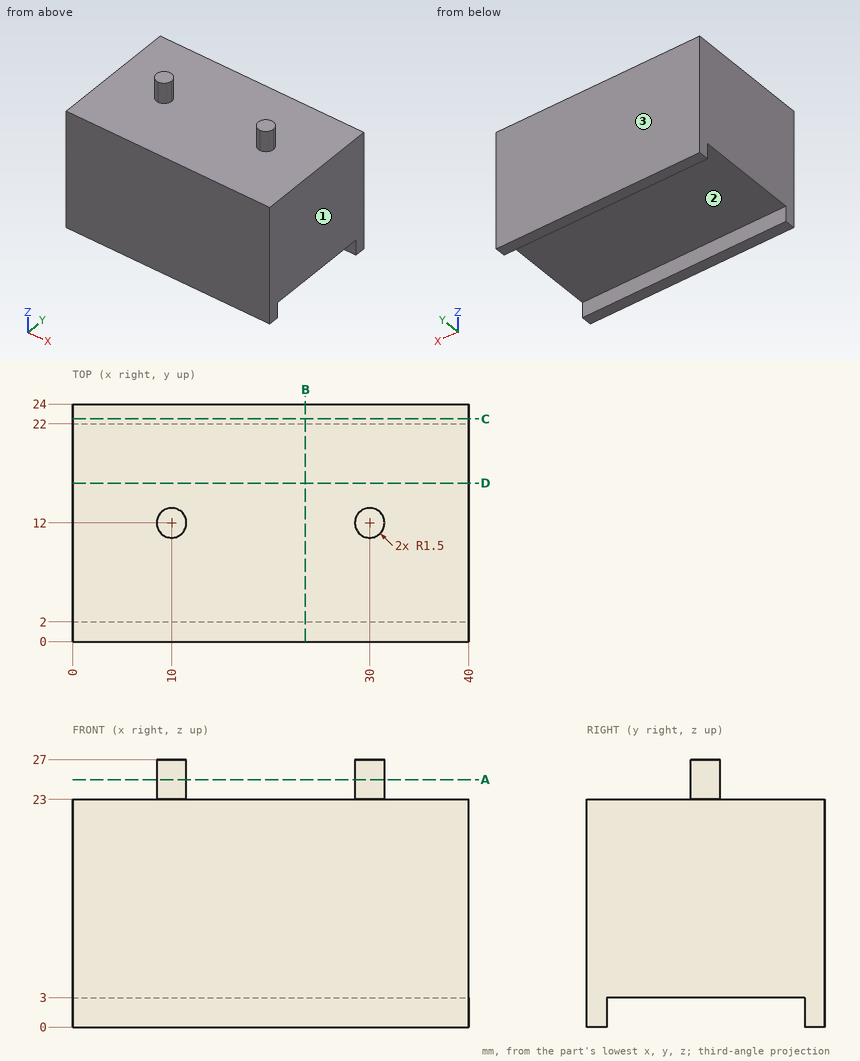
Drawing for the job (mm, zero at the part's lowest x, y, z). Round coordinates to 2 decimals unless told otherwise and drop trailing zeros. Write each loop counter-clockwise with the first axis right and the second up, starting at its lowest first coordinate (ties: lowest second). Pieces come first, ordered by that corner, then holes. Notation, with made-up numbers: (-14, -33) - (-9, -33) arc R12 cw to (-9, -26) - close; hole circle Ø8 at (-36.5, 51). An arc over 180 degrees is marked (long way). Return JSON: item names as keys, results as strings. Group by question number.
Item 1: Mould opens along Y. For the marked faces 1, 2 and 3 say: +Y half, -Y half, draft (parallel to the pull), parting line (faces both ways), or undercut.
Item 2: Flat gauge pins, fed straight in: pin 1 Ø1 at (x, y) = (30.5, 14) entering from +Z; pin 2 Ø3 at (x, z) = (33.5, 24) entering from +Y. Where does each tip first touch, or does it go through?
Item 3: Band-saw the part on A-A on z = 25. List the corners of the cut face in (x, y).
Item 4: Band-saw the part on D-D on y = 16. List the corners of the cut face in (x, z).
Item 5: Probe probe 1 along Z at (x, y) = (7, 5). List the from-to ranges inside material, lowest first.
Item 6: Band-saw the part on C-C on y = 22.5. List the corners of the cut face in (x, z).
Item 7: Band-saw the part on B-B on x = 23.5. List the corners of the cut face in (y, z).
Resolved:
{
 "1": {"face 1": "draft", "face 2": "undercut", "face 3": "+Y half"},
 "2": {"pin 1": "stops at z = 23", "pin 2": "stops at y = 24"},
 "3": {"outline": "circle Ø3 at (10, 12); circle Ø3 at (30, 12)"},
 "4": {"outline": "(0, 3) - (40, 3) - (40, 23) - (0, 23) - close"},
 "5": {"probe 1": "z = 3 to 23"},
 "6": {"outline": "(0, 0) - (40, 0) - (40, 23) - (0, 23) - close"},
 "7": {"outline": "(0, 0) - (2, 0) - (2, 3) - (22, 3) - (22, 0) - (24, 0) - (24, 23) - (0, 23) - close"}
}
